For this review, take the finished solid that the model builds, in its own axes (mm). Face numbers are marked on the shaded views. A direction names the side the tool comes from. Round coordinates to 2 decimals unless told otherwise and drop trailing zeros. Order: outer loops, then holes, each group sorted by start corner. A loop starts at its lowest first (then second) coordinate and runs counter-clockwise, first axis right, second up. Notation, with made-up numbers: M -1.75,42 L 20.25,42 A28 cw 20.25,70 Z; hole C 81,22 d11. An arc over 180 degrees is marked long. Answer as a JSON object with one key per item and string values.
from build123d import *

# Parameters (mm, degrees)
SKETCH_1_R          = 5.25
EXTRUDE_1_DEPTH     = 15
CUT_EXTRUDE_1_DEPTH = 10
EXTRUDE_2_DEPTH     = 18
SKETCH_4_R          = 1.5
CUT_EXTRUDE_2_DEPTH = 14.5
SKETCH_5_R          = 14
SKETCH_5_R_2        = 5.25
EXTRUDE_3_DEPTH     = 15
SKETCH_6_R          = 18.043638251
SKETCH_6_R_2        = 10
CUT_EXTRUDE_3_DEPTH = 15
SKETCH_7_R          = 6.986522344
EXTRUDE_4_DEPTH     = 15
SKETCH_8_R          = 1.35
CUT_EXTRUDE_4_DEPTH = 15


with BuildPart() as part:
    # 草图1 → 凸台-拉伸1 (new body)
    with BuildSketch(Plane.XY):
        with BuildLine():
            Line((-11.489125293, -8), (11.489125293, -8))
            ThreePointArc((11.489125293, -8), (0, 14), (-11.489125293, -8))
        make_face()
        Circle(SKETCH_1_R, mode=Mode.SUBTRACT)
    extrude(amount=EXTRUDE_1_DEPTH)

    # 草图2 → 切除-拉伸1 (cut)
    with BuildSketch(Plane.XY.offset(15)):
        with BuildLine():
            Line((-13.416407865, 4), (13.416407865, 4))
            ThreePointArc((13.416407865, 4), (0, 14), (-13.416407865, 4))
        make_face()
    extrude(amount=-CUT_EXTRUDE_1_DEPTH, mode=Mode.SUBTRACT)

    # 草图3 → 凸台-拉伸2 (add)
    with BuildSketch(Plane.XY.offset(15)):
        with BuildLine():
            Line((-7.123903424, 5.5), (7.123903424, 5.5))
            ThreePointArc((7.123903424, 5.5), (9, 0), (7.123903424, -5.5))
            Line((7.123903424, -5.5), (-7.123903424, -5.5))
            ThreePointArc((-7.123903424, -5.5), (-9, 0), (-7.123903424, 5.5))
        make_face()
    extrude(amount=EXTRUDE_2_DEPTH)

    # 草图4 → 切除-拉伸2 (cut, through all)
    with BuildSketch(Plane(origin=(0, 5.5, 0), x_dir=(1, 0, 0), z_dir=(0, 1, 0))):
        with Locations((4.5, -26.46)):
            Circle(SKETCH_4_R)
        with Locations((-4.5, -26.46)):
            Circle(SKETCH_4_R)
    extrude(amount=-CUT_EXTRUDE_2_DEPTH, mode=Mode.SUBTRACT)

    # 草图5 → 凸台-拉伸3 (add)
    with BuildSketch(Plane(origin=(0, 0, 0), x_dir=(-1, 0, 0), z_dir=(0, 0, -1))):
        Circle(SKETCH_5_R)
        Circle(SKETCH_5_R_2, mode=Mode.SUBTRACT)
    extrude(amount=-EXTRUDE_3_DEPTH)

    # 草图6 → 切除-拉伸3 (cut)
    with BuildSketch(Plane(origin=(0, 0, 0), x_dir=(-1, 0, 0), z_dir=(0, 0, -1))):
        Circle(SKETCH_6_R)
        Circle(SKETCH_6_R_2, mode=Mode.SUBTRACT)
    extrude(amount=-CUT_EXTRUDE_3_DEPTH, mode=Mode.SUBTRACT)

    # 草图7 → 凸台-拉伸4 (add)
    with BuildSketch(Plane(origin=(0, 0, 0), x_dir=(-1, 0, 0), z_dir=(0, 0, -1))):
        Circle(SKETCH_7_R)
        with BuildLine():
            Line((-1.985312345, 4.588957931), (3.849512157, 3.190808072))
            ThreePointArc((3.849512157, 3.190808072), (-1.165124883, -4.862353752), (-1.985312345, 4.588957931))
        make_face(mode=Mode.SUBTRACT)
    extrude(amount=-EXTRUDE_4_DEPTH)

    # 草图8 → 切除-拉伸4 (cut)
    with BuildSketch(Plane(origin=(-0.932099906, 3.889883001, 0), x_dir=(0.97247075, 0.233024977, 0), z_dir=(0.233024977, -0.97247075, 0))):
        with Locations((0, 7.544256547)):
            Circle(SKETCH_8_R)
    extrude(amount=-CUT_EXTRUDE_4_DEPTH, mode=Mode.SUBTRACT)


solid = part.part
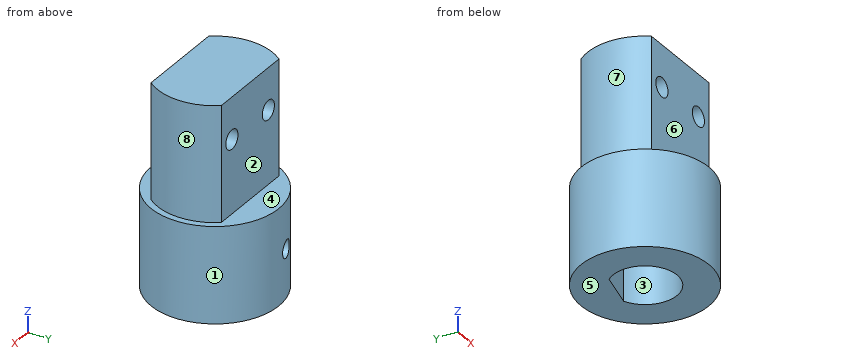
1) Mouldability with a two-part tool opening along Y and no side actions: class the marked faces 1, 2, 3 and 4 as +Y half, -Y half, draft (parallel to the pull), parting line (faces both ways), or undercut.
Geometry check:
{"face 1": "parting line", "face 2": "+Y half", "face 3": "undercut", "face 4": "draft"}
2) Add section B-B on x = -4.5. State the section outline as (y, z) points, and give its area (3 significant figures).
Geometry check:
{"outline": "M -8.93,0 L -2.18,0 L -2.18,15 L 2.18,15 L 2.18,0 L 8.93,0 L 8.93,15 L 5.5,15 L 5.5,24.96 L -5.5,24.96 L -5.5,15 L -8.93,15 Z; M -5.5,27.96 L 5.5,27.96 L 5.5,33 L -5.5,33 Z", "area": "368 mm²"}
3) Add section A-A on z = 26.46. State the section outline as (x, y) points, and give its area (3 significant figures).
Geometry check:
{"outline": "M -7.12,-5.5 L -6,-5.5 L -6,5.5 L -7.12,5.5 A9 ccw Z; M -3,-5.5 L 3,-5.5 L 3,5.5 L -3,5.5 Z; M 6,-5.5 L 7.12,-5.5 A9 ccw 7.12,5.5 L 6,5.5 Z", "area": "119 mm²"}
4) Add section D-D on x = -8. State the section outline as (y, z) points, and give its area (3 significant figures).
Geometry check:
{"outline": "M -6,0 L 6,0 L 6,15 L 4.12,15 L 4.12,33 L -4.12,33 L -4.12,15 L -6,15 Z", "area": "328 mm²"}
5) Machinability: for the marked faces 5, 6, 7 and 8, which of the approach directions +Z, -Z, +X, -X, +Y, -Y give a long, thin tool a straight path to every point of the face, cutting with its end or side? Answer none if there is none.
Geometry check:
{"face 5": "-Z, +X, -X, +Y, -Y", "face 6": "+Z, +X, -X, -Y", "face 7": "+Z, -X", "face 8": "+Z, +X"}
6) Add section C-C on y = 0. State the section outline as (x, z) points, and give its area (3 significant figures).
Geometry check:
{"outline": "M -10,0 L -5,0 L -5,15 L 5,15 L 5,0 L 10,0 L 10,15 L 9,15 L 9,33 L -9,33 L -9,15 L -10,15 Z; hole C -4.5,26.46 d3; hole C 4.5,26.46 d3", "area": "460 mm²"}
7) For L1, parallel to Z at x = 4.5, y = -3; L2, parallel to X at y = 0, z = 4.5; L3, parallel to Y at x = -3.75, z = 18.5, list the stretches that pass through material, from the lowest coordinate up.
Geometry check:
{"L1": "z = 0 to 24.96, 27.96 to 33", "L2": "x = -10 to -5, 5 to 10", "L3": "y = -5.5 to 5.5"}
8) Insertion check: P1, Ø2, axis at x = 0.5, y = 3, coming from the -Z side; P2, Ø3.5, axis at x = -4.5, z = 26.46, coming from the -Y side; P3, Ø5, axis at y = -7, z = 7.5, coming from the -X side. Each pin has a flat end and moves straight along its axis. Give the tip position at first contact, or say it passes through.
Geometry check:
{"P1": "stops at z = 15", "P2": "stops at y = -5.5", "P3": "stops at x = -8.93"}
